from build123d import *

# Parameters (mm, degrees)
BOSS_EXTRUDE1_DEPTH = 457.2
FILLET1_R           = 0.508


with BuildPart() as part:
    # Sketch1 → Boss-Extrude1 (new body, symmetric)
    with BuildSketch(Plane.XY):
        Polygon((7.332348419, 0), (3.666174209, 6.35), (-3.666174209, 6.35), (-7.332348419, 0), (-3.666174209, -6.35), (3.666174209, -6.35), align=None)
    extrude(amount=BOSS_EXTRUDE1_DEPTH, both=True)

    # Fillet1
    fillet1_edges = [part.edges().sort_by_distance(p)[0] for p in [
        (3.666174209, -6.35, 0),
        (-3.666174209, -6.35, 0),
        (-7.332348419, 0, 0),
        (-3.666174209, 6.35, 0),
        (3.666174209, 6.35, 0),
        (7.332348419, 0, 0),
    ]]
    fillet(fillet1_edges, radius=FILLET1_R)


solid = part.part
Could you check a few things on this model? Use its own coordinates, in mm. Give positions to 0.01 mm unless a question says otherwise; leave off trailing zeros. Order: outer loops, then holes, each group sorted by start corner. A loop starts at its lowest first (then second) coordinate and runs counter-clockwise, first axis right, second up. Notation, with made-up numbers: (59.25, 7.5) -> (101.25, 7.5) arc R11 ccw to (101.25, 25.5) -> close; hole circle Ø2 at (17.25, 21). An arc over 180 degrees is marked (long way). Answer in a Markdown table with one row per item. Add a question column.
Item 1: Imagine slicing it at A-A (z = -318). List the corners of the cut face in (x, y) for me.
Item 2: Please list where these lines run through material, in increasing order: probe 1 along X at (y, z) = (-1.5, -112); probe 2 along X at (y, z) = (-0.5, 58); probe 3 along Y at (x, z) = (4.25, 209.5).
Item 3: Imagine slicing it at B-B (y = -2.5). List the corners of the cut face in (x, z) for me.
Item 4: I'm going to push a flat-ended pin straight in: P1, Ø6, axis at y = -0.5, z = 92.5, coming from the -X side. Where does the tip first touch, or does it pass through?
Result:
| question | item | result |
|---|---|---|
| 1 | outline | (-7.19, -0.25) -> (-3.81, -6.1) arc R0.51 ccw to (-3.37, -6.35) -> (3.37, -6.35) arc R0.51 ccw to (3.81, -6.1) -> (7.19, -0.25) arc R0.51 ccw to (7.19, 0.25) -> (3.81, 6.1) arc R0.51 ccw to (3.37, 6.35) -> (-3.37, 6.35) arc R0.51 ccw to (-3.81, 6.1) -> (-7.19, 0.25) arc R0.51 ccw to start |
| 2 | probe 1 | -6.47 to 6.47 |
| 2 | probe 2 | -7.04 to 7.04 |
| 2 | probe 3 | -5.34 to 5.34 |
| 3 | outline | (-5.89, -457.2) -> (5.89, -457.2) -> (5.89, 457.2) -> (-5.89, 457.2) -> close |
| 4 | P1 | x = -7.25 |
